Check sheet for the modelled part. Datum: model origin and axes. Units: mm. Face numbers are marked on the shaded views. A direction names the side the tool comes from. Round coordinates to 2 decimals unless told otherwise and drop trailing zeros. Loops run counter-clockwise (first coordinate to the right, second up) from the corner with the lowest first, then second, coordinate; pieces in that order, holes last. Notation, with made-up numbers: (52, 75.5) - (86, 75.5) arc R10 cw to (86, 84.5) - close; hole circle Ø2 at (-8, -11.5). An arc over 180 degrees is marked (long way). Answer in a Markdown table with one row per item. Add a question column.
(1) Thickness scan on line 1 along Y through (x, z) = (0, 0.25); line 2 along Y through (x, z) = (0, -8.5); line 3 along Z through (x, y) = (0.5, -11.25). Record the ranges inside material, lowest first.
(2) Access from +Z, -Z, +X, -X, +Y, -Y to the whole of each face (thin tool, end or side, straight path). Record for the marked faces 1, 2 and 3.
(3) Cross-section at C-C on z = 4.75. Enter the section's corners in (x, y), then the cut area to 3 significant figures.
(4) Gauge pin test, flat ends, axial feed: pin 1 (5 mm diameter, centred on x = -8, z = -10.5, fed in from -Y); pin 2 (6 mm diameter, centred on x = 7, z = -10, fed in from +Y); pin 3 (8 mm diameter, centred on y = 7.5, z = -10, fed in from +X). Record the tip position at first contact, or that the pin passes through.
(5) Cross-section at A-A on x = 0. Enter the section's corners in (y, z).
(6) Cross-section at D-D on x = -9. Enter the section's corners in (y, z), then the cut area to 3 significant figures.
from build123d import *

# Parameters (mm, degrees)
CUT_EXTRUDE1_DEPTH      = 30.444863729
CUT_EXTRUDE1_DEPTH_BACK = 30.444863729
SKETCH3_R               = 7


with BuildPart() as part:
    # Sketch2 → Revolve1 (revolve)
    with BuildSketch(Plane.YZ, mode=Mode.PRIVATE) as revolve1_sk:
        Polygon((0, 7), (10, 7), (10, 3), (13, 3), (13, 0), (10, 0), (10, -13), (9.5, -13), (9.5, -14.35), (10, -14.35), (10, -16), (0, -16), align=None)
    revolve(revolve1_sk.sketch.rotate(Axis((0, 0, 15.904017857), (0, 0, -1)), 90), axis=Axis((0, 0, 15.904017857), (0, 0, -1)))

    # Sketch3 → Cut-Extrude1 (cut, two sides: drawn at the far end of the back side and taken through both)
    with BuildSketch(Plane.XY.offset(7).offset(-CUT_EXTRUDE1_DEPTH_BACK)):
        Circle(SKETCH3_R)
    extrude(amount=CUT_EXTRUDE1_DEPTH + CUT_EXTRUDE1_DEPTH_BACK, mode=Mode.SUBTRACT)


solid = part.part
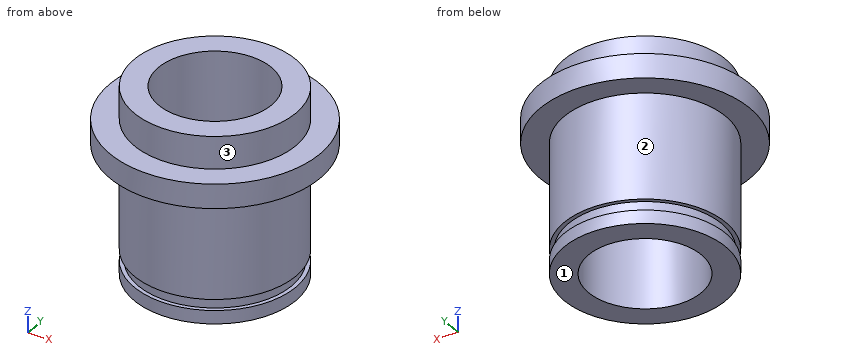
Answers:
| question | item | result |
|---|---|---|
| 1 | line 1 | y = -13 to -7, 7 to 13 |
| 1 | line 2 | y = -10 to -7, 7 to 10 |
| 1 | line 3 | z = 0 to 3 |
| 2 | face 1 | -Z, +X, -X, +Y, -Y |
| 2 | face 2 | -Z |
| 2 | face 3 | +Z |
| 3 | outline | circle Ø20 at (0, 0); hole circle Ø14 at (0, 0) |
| 3 | area | 160 mm^2 |
| 4 | pin 1 | stops at y = -8.35 |
| 4 | pin 2 | stops at y = 9.17 |
| 4 | pin 3 | stops at x = 9.37 |
| 5 | outline | (-13, 0) - (-10, 0) - (-10, -13) - (-9.5, -13) - (-9.5, -14.35) - (-10, -14.35) - (-10, -16) - (-7, -16) - (-7, 7) - (-10, 7) - (-10, 3) - (-13, 3) - close; (7, -16) - (10, -16) - (10, -14.35) - (9.5, -14.35) - (9.5, -13) - (10, -13) - (10, 0) - (13, 0) - (13, 3) - (10, 3) - (10, 7) - (7, 7) - close |
| 6 | outline | (-9.38, 0) - (-4.36, 0) - (-4.36, -13) - (-3.04, -13) - (-3.04, -14.35) - (-4.36, -14.35) - (-4.36, -16) - (4.36, -16) - (4.36, -14.35) - (3.04, -14.35) - (3.04, -13) - (4.36, -13) - (4.36, 0) - (9.38, 0) - (9.38, 3) - (4.36, 3) - (4.36, 7) - (-4.36, 7) - (-4.36, 3) - (-9.38, 3) - close |
| 6 | area | 227 mm^2 |
